Read the model definition and answer for the solid it produces. Units are mm, in the model's axes. A direction names the side the tool comes from. Coordinates: 2 decimals unless noted, no trailing zeros. Write each loop counter-clockwise with the first axis right and the second up, starting at its lowest first coordinate (ties: lowest second). Pieces come first, ordered by that corner, then holes.
1) Which of the six approach directions +Z, -Z, +X, -X, +Y, -Y give full straight-line access (tool end or side, diameter ignored) to faces 1 (the face through (-23.016, -7.248, 1.288)), 2 (the face through (0, 0, 133.811)), 3 (the face through (0.34, 1.55, 129.95))?
2) Find the intervals of material crossed by line 1 (X direction, y = 0, z = 1.6); line 2 (Y direction, x = -0.5, z = 81), in increasing order.
3) Each of these flat-tipped pins is pushed along its axis until it touches: pin 1 Ø1 at (y, z) = (18, 30.5) entering from +X; pin 2 Ø10 at (x, y) = (-17.5, 11.5) entering from +Z; pin 3 Ø1 at (x, z) = (-17, 30) entering from +Y. Where does it stop, or does it pass through?
4) The part is cut by section A-A (z = 97.5). Determine the outline of the cut face in (x, y).
from build123d import *


with BuildPart() as f1:
    # F0 (on Front) → F1 (revolve)
    with BuildSketch(Plane.XZ):
        with BuildLine():
            Line((-26.67, 99.568), (-26.67, 0))
            Line((-26.67, 0), (-24.13, 0))
            Line((-24.13, 0), (-24.13, 2.54))
            ThreePointArc((-24.13, 2.54), (-12.965124, 9.757795), (0, 12.7))
            Line((0, 12.7), (0, 133.810711))
            Line((0, 133.810711), (-1.5875, 133.810711))
            Line((-1.5875, 133.810711), (-1.5875, 126.190711))
            ThreePointArc((-1.5875, 126.190711), (-19.411691, 117.856661), (-26.67, 99.568))
        make_face()
    revolve(axis=Axis((0, 0, 73.255356), (0, 0, 1)))


with BuildPart() as f3:
    # F2 (on Front) → F3 (revolve)
    with BuildSketch(Plane.XZ):
        Polygon((-9.525, 133.810711), (0, 133.810711), (0, 151.590711), (-1.5875, 151.590711), (-1.5875, 138.890711), (-12.065, 138.890711), (-12.065, 121.110711), (-9.525, 121.110711), align=None)
    revolve(axis=Axis((0, 0, 142.700711), (0, 0, -1)))


solid = f1.part
Reported:
1. face 1: -Z
1. face 2: +Z, +X, -X, +Y, -Y
1. face 3: +Z
2. line 1: x = -26.67 to -24.13, 24.13 to 26.67
2. line 2: y = -26.67 to 26.67
3. pin 1: stops at x = 20.13
3. pin 2: stops at z = 120.95
3. pin 3: stops at y = 20.95
4. outline: circle Ø53.34 at (0, 0)
